CAD build for the part. Positions are in the model's coordinates, mm. Face numbers are marked on the shaded views. Give positions to 0.01 mm unless a question says otherwise; leave off trailing zeros. Loops run counter-clockwise (first coordinate to the right, second up) from the corner with the lowest first, then second, coordinate; pieces in that order, holes last.
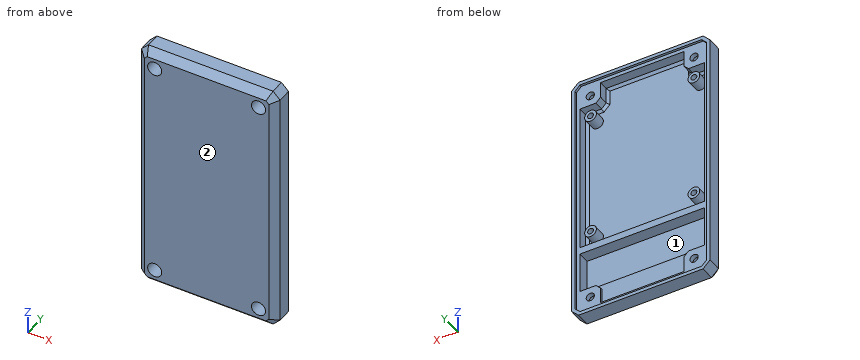
Autodesk Inventor part; units mm, degrees
ref_plane "YZ Plane" through (0, 0, 0) normal (1, 0, 0) x (0, 1, 0)
ref_plane "XZ Plane" through (0, 0, 0) normal (0, 1, 0) x (-1, 0, 0)
ref_plane "XY Plane" through (0, 0, 0) normal (0, 0, 1) x (1, 0, 0)
sketch "Sketch4" plane through (0, 0, 0) normal (0, 1, 0) x (-1, 0, 0)
  circle A0 centre (-31.1, -7.3) radius 1.75
  line L0 (-34.858, -107.35) -> (16.858, -107.35)
  line L1 (16.858, -107.35) -> (18.95, -105.258)
  line L2 (18.95, -105.258) -> (18.95, -3.542)
  line L3 (18.95, -3.542) -> (16.858, -1.45)
  line L4 (16.858, -1.45) -> (-34.858, -1.45)
  line L5 (-34.858, -1.45) -> (-36.95, -3.542)
  line L6 (-36.95, -3.542) -> (-36.95, -105.258)
  line L7 (-36.95, -105.258) -> (-34.858, -107.35)
  circle A1 centre (-31.1, -101.5) radius 1.75
  circle A2 centre (13.1, -7.3) radius 1.75
  line L8 (8.7, -99.1) -> (10.7, -97.1)
  line L9 (8.7, -99.1) -> (8.7, -105.9)
  line L10 (8.7, -105.9) -> (-26.7, -105.9)
  line L11 (-26.7, -99.1) -> (-26.7, -105.9)
  line L12 (-28.7, -97.1) -> (-26.7, -99.1)
  line L13 (-35.5, -97.1) -> (-28.7, -97.1)
  line L14 (-35.5, -97.1) -> (-35.5, -11.7)
  line L15 (-35.5, -11.7) -> (-28.7, -11.7)
  line L16 (-26.7, -9.7) -> (-28.7, -11.7)
  line L17 (-26.7, -9.7) -> (-26.7, -2.9)
  line L18 (-26.7, -2.9) -> (8.7, -2.9)
  line L19 (8.7, -9.7) -> (8.7, -2.9)
  line L20 (10.7, -11.7) -> (8.7, -9.7)
  line L21 (17.5, -11.7) -> (10.7, -11.7)
  line L22 (17.5, -11.7) -> (17.5, -97.1)
  line L23 (17.5, -97.1) -> (10.7, -97.1)
  circle A3 centre (13.1, -101.5) radius 1.75
  line L24 (20.5, -2.9) -> (20.5, -105.9)
  line L25 (17.5, 0.1) -> (20.5, -2.9)
  line L26 (-35.5, 0.1) -> (17.5, 0.1)
  line L27 (-38.5, -2.9) -> (-35.5, 0.1)
  line L28 (-38.5, -105.9) -> (-38.5, -2.9)
  line L29 (-35.5, -108.9) -> (-38.5, -105.9)
  line L30 (17.5, -108.9) -> (-35.5, -108.9)
  line L31 (20.5, -105.9) -> (17.5, -108.9)
  line L32 (16.858, -107.35) -> (18.95, -105.258)
  line L33 (-34.858, -107.35) -> (16.858, -107.35)
  line L34 (-36.95, -105.258) -> (-34.858, -107.35)
  line L35 (-36.95, -3.542) -> (-36.95, -105.258)
  line L36 (-34.858, -1.45) -> (-36.95, -3.542)
  line L37 (16.858, -1.45) -> (-34.858, -1.45)
  line L38 (18.95, -3.542) -> (16.858, -1.45)
  line L39 (18.95, -105.258) -> (18.95, -3.542)
  line L40 (-37.05, -105.2994) -> (-37.05, -3.5006)
  line L41 (-37.05, -3.5006) -> (-34.8994, -1.35)
  line L42 (-34.8994, -1.35) -> (16.8994, -1.35)
  line L43 (16.8994, -1.35) -> (19.05, -3.5006)
  line L44 (19.05, -3.5006) -> (19.05, -105.2994)
  line L45 (19.05, -105.2994) -> (16.8994, -107.45)
  line L46 (16.8994, -107.45) -> (-34.8994, -107.45)
  line L47 (-34.8994, -107.45) -> (-37.05, -105.2994)
  point P0 (0, 0)
  point P1 (0, 0)
  dimension "d29" = 0.1
extrude "Extrusion3" add sketch "Sketch4" along normal blind 1 contours L24 L31 L30 L29 L28 L27 L26 L25
extrude "Extrusion4" add sketch "Sketch4" against normal blind 5 contours L7 L6 L5 L4 L3 L2 L1 L0 | L24 L31 L30 L29 L28 L27 L26 L25 | L40 L41 L42 L43 L44 L45 L46 L47
sketch "Sketch5" plane through (0, -5, 0) normal (0, -1, 0) x (1, 0, 0)
  line L0 (38.5, -105.9) -> (38.5, -2.9)
  line L1 (38.5, -2.9) -> (35.5, 0.1)
  line L2 (35.5, 0.1) -> (-17.5, 0.1)
  line L3 (35.5, 0.1) -> (-17.5, 0.1)
  line L4 (-17.5, 0.1) -> (-20.5, -2.9)
  line L5 (-20.5, -2.9) -> (-20.5, -105.9)
  line L6 (-20.5, -105.9) -> (-17.5, -108.9)
  line L7 (-17.5, -108.9) -> (35.5, -108.9)
  line L8 (35.5, -108.9) -> (38.5, -105.9)
  line L9 (38.5, -105.9) -> (38.5, -2.9)
  line L10 (38.5, -2.9) -> (35.5, 0.1)
  circle A0 centre (31.1, -101.5) radius 1.75
  circle A1 centre (-13.1, -101.5) radius 1.75
  circle A2 centre (31.1, -7.3) radius 1.75
  circle A3 centre (-13.1, -7.3) radius 1.75
  line L11 (-17.5, -11.7) -> (-10.7, -11.7)
  line L12 (-10.7, -11.7) -> (-8.7, -9.7)
  line L13 (-8.7, -9.7) -> (-8.7, -2.9)
  line L14 (-8.7, -2.9) -> (26.7, -2.9)
  line L15 (26.7, -2.9) -> (26.7, -9.7)
  line L16 (26.7, -9.7) -> (28.7, -11.7)
  line L17 (28.7, -11.7) -> (35.5, -11.7)
  line L18 (35.5, -11.7) -> (35.5, -97.1)
  line L19 (35.5, -97.1) -> (28.7, -97.1)
  line L20 (28.7, -97.1) -> (26.7, -99.1)
  line L21 (26.7, -99.1) -> (26.7, -105.9)
  line L22 (26.7, -105.9) -> (-8.7, -105.9)
  line L23 (-8.7, -105.9) -> (-8.7, -99.1)
  line L24 (-8.7, -99.1) -> (-10.7, -97.1)
  line L25 (-10.7, -97.1) -> (-17.5, -97.1)
  line L26 (-17.5, -97.1) -> (-17.5, -11.7)
  point P0 (0, 0)
extrude "Extrusion5" add sketch "Sketch5" along normal blind 3 contours L8 L7 L6 L5 L4 L2 L1 L0 | L11 L12 L13 L14 L15 L16 L17 L18 L19 L20 L21 L22 L23 L24 L25 L26
sketch "Sketch6" plane through (0, -8, 0) normal (0, -1, 0) x (1, 0, 0)
  line L0 (38.5, -2.9) -> (35.5, 0.1)
  line L1 (35.5, 0.1) -> (-17.5, 0.1)
  line L2 (-17.5, 0.1) -> (-20.5, -2.9)
  line L3 (-20.5, -2.9) -> (-20.5, -105.9)
  line L4 (-20.5, -105.9) -> (-17.5, -108.9)
  line L5 (-17.5, -108.9) -> (35.5, -108.9)
  line L6 (35.5, -108.9) -> (38.5, -105.9)
  line L7 (38.5, -105.9) -> (38.5, -2.9)
  circle A0 centre (31.1, -101.5) radius 1.75
  circle A1 centre (-13.1, -101.5) radius 1.75
  circle A2 centre (31.1, -7.3) radius 1.75
  circle A3 centre (-13.1, -7.3) radius 1.75
  circle A4 centre (31.1, -7.3) radius 3
  circle A5 centre (31.1, -101.5) radius 3
  circle A6 centre (-13.1, -101.5) radius 3
  circle A7 centre (-13.1, -7.3) radius 3
  point P0 (0, 0)
  dimension "d17" = 6
  dimension "d18" = 6
  dimension "d19" = 6
  dimension "d20" = 6
extrude "Extrusion6" cut sketch "Sketch6" against normal blind 6 contours A4 | A5 | A6 | A7
chamfer "Chamfer2" distance 1 angle 45 16 edges at (-17.5, -5, -54.4) (-9.7, -5, -98.1) (-8.7, -5, -102.5) (9, -5, -105.9) (26.7, -5, -102.5) (27.7, -5, -98.1) (35.5, -5, -54.4) (-14.1, -5, -11.7) (-9.7, -5, -10.7) (-8.7, -5, -6.3) (9, -5, -2.9) (26.7, -5, -6.3) (27.7, -5, -10.7) (32.1, -5, -11.7) (32.1, -5, -97.1) (-14.1, -5, -97.1)
chamfer "Chamfer3" distance 3 angle 45 8 edges at (38.5, -8, -54.4) (37, -8, -1.4) (9, -8, 0.1) (-19, -8, -1.4) (-20.5, -8, -54.4) (-19, -8, -107.4) (9, -8, -108.9) (37, -8, -107.4)
sketch "Sketch7" plane through (0, -5, 0) normal (0, 1, 0) x (1, 0, 0)
  line L0 (-13, 16.7) -> (31, 16.7) construction
  line L1 (31, 16.7) -> (31, 70.7) construction
  line L2 (31, 70.7) -> (-13, 70.7) construction
  line L3 (-13, 70.7) -> (-13, 16.7) construction
  circle A0 centre (-13, 70.7) radius 1.25
  circle A1 centre (31, 70.7) radius 1.25
  circle A2 centre (31, 16.7) radius 1.25
  circle A3 centre (-13, 16.7) radius 1.25
  line L4 (-13, 70.7) -> (31, 16.7) construction
  line L5 (-13, 16.7) -> (31, 70.7) construction
  line L6 (-16, 13.7) -> (34, 13.7) construction
  line L7 (34, 13.7) -> (34, 73.7) construction
  line L8 (34, 73.7) -> (-16, 73.7) construction
  line L9 (-16, 73.7) -> (-16, 13.7) construction
  line L10 (-16, 13.7) -> (34, 73.7) construction
  line L11 (34, 13.7) -> (-16, 73.7) construction
  line L12 (34.5, 96.1) -> (34.5, 12.7) construction
  line L13 (25.7, 98.6858) -> (28.2858, 96.1) construction
  line L14 (25.7, 104.9) -> (25.7, 98.6858) construction
  line L15 (-7.7, 104.9) -> (25.7, 104.9) construction
  line L16 (-7.7, 98.6858) -> (-7.7, 104.9) construction
  line L17 (-10.2858, 96.1) -> (-7.7, 98.6858) construction
  line L18 (-16.5, 12.7) -> (-16.5, 96.1) construction
  line L19 (-10.2858, 12.7) -> (-16.5, 12.7) construction
  line L20 (-7.7, 10.1142) -> (-10.2858, 12.7) construction
  line L21 (-7.7, 3.9) -> (-7.7, 10.1142) construction
  line L22 (25.7, 3.9) -> (-7.7, 3.9) construction
  line L23 (25.7, 10.1142) -> (25.7, 3.9) construction
  line L24 (28.2858, 12.7) -> (25.7, 10.1142) construction
  line L25 (34.5, 12.7) -> (28.2858, 12.7) construction
  line L26 (-7.7, 104.9) -> (25.7, 104.9) construction
  line L27 (9, 104.9) -> (9, 3.9) construction
  line L28 (25.7, 3.9) -> (-7.7, 3.9) construction
  circle A4 centre (-13, 70.7) radius 2.5
  circle A5 centre (31, 70.7) radius 2.5
  circle A6 centre (31, 16.7) radius 2.5
  circle A7 centre (-13, 16.7) radius 2.5
  line L29 (28.2858, 96.1) -> (34.5, 96.1)
  line L30 (-16.5, 96.1) -> (-10.2858, 96.1)
  point P0 (0, 0)
  point P1 (9, 43.7)
  point P2 (9, 43.7)
  dimension "d30" = 44
  dimension "d31" = 54
  dimension "d32" = 2.5
  dimension "d33" = 2.5
  dimension "d34" = 2.5
  dimension "d35" = 2.5
  dimension "d36" = 50
  dimension "d37" = 60
  dimension "d38" = 1
  dimension "d39" = 5
  dimension "d40" = 5
  dimension "d41" = 5
  dimension "d42" = 5
extrude "Extrusion7" add sketch "Sketch7" along normal blind 5
sketch "Sketch8" plane through (0, -5, 0) normal (0, 1, 0) x (1, 0, 0)
  line L0 (-14.5, 79.6) -> (35.5, 79.6)
  line L1 (35.5, 79.6) -> (35.5, 97.1)
  line L2 (35.5, 97.1) -> (-14.5, 97.1)
  line L3 (-14.5, 97.1) -> (-14.5, 79.6)
  line L4 (-14.5, 79.6) -> (35.5, 97.1) construction
  line L5 (35.5, 79.6) -> (-14.5, 97.1) construction
  circle A0 centre (31, 16.7) radius 2.5
  circle A1 centre (31, 70.7) radius 2.5
  circle A2 centre (-13, 16.7) radius 2.5
  circle A3 centre (-13, 70.7) radius 2.5
  line L6 (-16.5, 12.7) -> (-16.5, 96.1)
  line L7 (-10.2858, 12.7) -> (-16.5, 12.7)
  line L8 (-7.7, 10.1142) -> (-10.2858, 12.7)
  line L9 (-7.7, 3.9) -> (-7.7, 10.1142)
  line L10 (25.7, 3.9) -> (-7.7, 3.9)
  line L11 (25.7, 10.1142) -> (25.7, 3.9)
  line L12 (28.2858, 12.7) -> (25.7, 10.1142)
  line L13 (34.5, 12.7) -> (28.2858, 12.7)
  line L14 (34.5, 96.1) -> (34.5, 12.7)
  line L15 (25.7, 98.6858) -> (28.2858, 96.1)
  line L16 (25.7, 104.9) -> (25.7, 98.6858)
  line L17 (-7.7, 104.9) -> (25.7, 104.9)
  line L18 (-7.7, 98.6858) -> (-7.7, 104.9)
  line L19 (-10.2858, 96.1) -> (-7.7, 98.6858)
  line L20 (28.7, 97.1) -> (35.5, 97.1)
  line L21 (35.5, 97.1) -> (35.5, 11.7)
  line L22 (28.2858, 96.1) -> (34.5, 96.1)
  line L23 (-16.5, 96.1) -> (-10.2858, 96.1)
  line L24 (26.7, 105.9) -> (-8.7, 105.9)
  line L25 (-7.7, 104.9) -> (-8.7, 105.9)
  line L26 (-7.7, 104.9) -> (25.7, 104.9)
  line L27 (25.7, 104.9) -> (26.7, 105.9)
  line L28 (-8.7, 105.9) -> (-8.7, 99.1)
  line L29 (-7.7, 98.6858) -> (-8.7, 99.1)
  line L30 (-7.7, 98.6858) -> (-7.7, 104.9)
  line L31 (-7.7, 104.9) -> (-8.7, 105.9)
  line L32 (-8.7, 99.1) -> (-10.7, 97.1)
  line L33 (-10.2858, 96.1) -> (-10.7, 97.1)
  line L34 (-10.2858, 96.1) -> (-7.7, 98.6858)
  line L35 (-7.7, 98.6858) -> (-8.7, 99.1)
  line L36 (28.7, 97.1) -> (26.7, 99.1)
  line L37 (25.7, 98.6858) -> (26.7, 99.1)
  line L38 (25.7, 98.6858) -> (28.2858, 96.1)
  line L39 (28.2858, 96.1) -> (28.7, 97.1)
  line L40 (26.7, 99.1) -> (26.7, 105.9)
  line L41 (25.7, 104.9) -> (26.7, 105.9)
  line L42 (25.7, 104.9) -> (25.7, 98.6858)
  line L43 (25.7, 98.6858) -> (26.7, 99.1)
  point P0 (0, 0)
  point P1 (10.5, 88.35)
  point P2 (34.5, 97.1)
  point P3 (-9.2858, 97.1)
  point P4 (-14.5, 96.1)
  dimension "d47" = 50
  dimension "d48" = 17.5
extrude "Extrusion8" cut sketch "Sketch8" along normal blind 5 contours L3 L23 L19 L2 L15 L22 L14 L0 | L14 L22 L39 L2 L1 L0 | L3 L2 L33 L23 | L33 L2 L19 | L15 L2 L39
extrude "Extrusion9" add sketch "Sketch8" along normal blind 4 contours L32 L29 L19 L2 | L19 L18 L17 L16 L15 L2 | L2 L15 L37 L36 | L28 L25 L18 L29 | L37 L16 L27 L40 | L24 L27 L17 L25
sketch "Sketch9" plane through (0, -5, 0) normal (0, 1, 0) x (1, 0, 0)
  line L0 (34.5, 79.6) -> (35.5, 79.6)
  line L1 (-17.5, 97.1) -> (-17.5, 11.7)
  line L2 (35.5, 79.6) -> (-17.5, 79.6)
  line L3 (-17.5, 79.6) -> (-17.5, 76.6)
  line L4 (-17.5, 76.6) -> (35.5, 76.6)
  line L5 (35.5, 76.6) -> (35.5, 79.6)
  point P0 (0, 0)
  dimension "d53" = 3
extrude "Extrusion10" add sketch "Sketch9" along normal blind 5
equation "\"d18\" = d17"
equation "\"d19\" = d17"
equation "\"d20\" = d17"
equation "\"d33\" = d32"
equation "\"d34\" = d32"
equation "\"d35\" = d32"
equation "\"d43\" = d42"
properties part number "_3DPrint"
1. Probe line 1 along Z through (x, y) = (20.5, -2); line 2 along X through (y, z) = (-2.7, -70.7); line 3 along Z through (x, y) = (21, -0.75). List the from-to ranges inside material, lowest first.
Responses:
line 1: z = -108.9 to -97.1, -79.6 to -76.6, -2.9 to 0.1
line 2: x = -20.5 to -17.5, -15.5 to -14.25, -11.75 to -10.5, 28.5 to 29.75, 32.25 to 33.5, 35.5 to 38.5
line 3: z = -108.9 to -105.9, -79.6 to -76.6, -2.9 to 0.1
2. Drop flat-ended pins along their axis: pin 1 (5 mm diameter, centred on x = 31.1, z = -101.5, fed in from +Y); pin 2 (1.5 mm diameter, centred on x = 12.5, z = -40.5, fed in from +Y). Give the stop position or say it passes through.
Responses:
pin 1: stops at y = 0
pin 2: stops at y = -5
3. Pull direction Z, two halves, no side cores. Call the marked faces 1 and 2: released by +Z, released by -Z, zero draft, split by the parting line, or undercut.
Responses:
face 1: undercut
face 2: zero draft
4. Saw through at D-D, the plane x = 11. List the corners of the cut face in (y, z), and give its area (3 significant figures).
Responses:
outline: (-8, -105.9) - (-5, -108.9) - (1, -108.9) - (1, -107.45) - (0, -107.45) - (0, -105.9) - (-1, -105.9) - (-1, -97.1) - (-5, -97.1) - (-5, -79.6) - (0, -79.6) - (0, -76.6) - (-5, -76.6) - (-5, -3.9) - (-4, -2.9) - (0, -2.9) - (0, -1.35) - (1, -1.35) - (1, 0.1) - (-5, 0.1) - (-8, -2.9) - close
area: 402 mm2
5. Saw through at A-A, the plane z = -7.3. Count the separate pieces of the cut face and the enclosed holes in it, and give its area (3 significant figures).
Responses:
separate pieces: 3
enclosed holes: 0
area: 204 mm2
